The listing builds one solid part. Answer for the finished solid, in the listing's coordinates (mm). Round coordinates to 2 decimals unless told otherwise and drop trailing zeros. Order: outer loops, then holes, each group sorted by start corner. A loop starts at its lowest first (then second) coordinate and runs counter-clockwise, first axis right, second up. Notation, with made-up numbers: (46.25, -37.5) -> (65.25, -37.5) arc R20 ccw to (65.25, -22.5) -> close; hole circle Ø8 at (11.25, -12). An arc over 180 degrees is marked (long way). Return JSON: item names as keys, results as strings. Group by question number.
(1) The part is cut by section B-B (z = -63.5). Determine the outline of the cut face in (x, y).
(2) The part is cut by section A-A (x = -12.7). Determine the outline of the cut face in (y, z).
(3) The part is cut by section D-D (x = -63.5). Determine the outline of the cut face in (y, z), plus the area to 3 significant figures.
(4) The part is cut by section C-C (y = 2). Determine the outline of the cut face in (x, z).
(5) Consider line 1 (Z direction, x = -12.7, y = 4.5); line 2 (Z direction, x = -63.5, y = 5); line 3 (Z direction, x = -51, y = 3.5). Determine where each line is inside the solid, lowest interval first. Write a range as [from, to].
(6) Each of these flat-tipped pins is pushed along its axis until it touches: pin 1 (3 mm diameter, centred on x = -38, y = 0.5, fed in from -Z); pin 2 (4.5 mm diameter, centred on x = -12.7, z = -12.7, fed in from +Y); pin 3 (2 mm diameter, centred on x = -56.5, y = 3.5, fed in from -Z). Where does it stop, or does it pass through?
Autodesk Inventor part; units mm, degrees
ref_plane "YZ Plane" through (0, 0, 0) normal (1, 0, 0) x (0, 1, 0)
ref_plane "XZ Plane" through (0, 0, 0) normal (0, 1, 0) x (-1, 0, 0)
ref_plane "XY Plane" through (0, 0, 0) normal (0, 0, 1) x (1, 0, 0)
sketch "Sketch1" plane through (0, 0, 0) normal (0, 1, 0) x (-1, 0, 0)
  line L0 (0, 0) -> (76.2, 0)
  line L1 (76.2, 0) -> (76.2, -25.4)
  line L2 (76.2, -25.4) -> (50.8, -25.4)
  line L3 (0, -25.4) -> (0, 0)
  line L4 (0, 0) -> (25.4, 0)
  line L5 (25.4, -50.8) -> (25.4, -76.2)
  line L6 (25.4, -76.2) -> (0, -76.2)
  line L7 (0, -76.2) -> (0, 0)
  arc A0 (50.8, -25.4) -> (25.4, -50.8) centre (50.8, -50.8) ccw
  circle A1 centre (63.5, -12.7) radius 2.5
  circle A2 centre (38.1, -12.7) radius 2.5
  circle A3 centre (12.7, -12.7) radius 2.5
  circle A4 centre (12.7, -38.1) radius 2.5
  circle A5 centre (12.7, -63.5) radius 2.5
  point P0 (12.7, -76.2)
  point P1 (76.2, -12.7)
  dimension "d0" = 76.2
  dimension "d1" = 25.4
  dimension "d2" = 25.4
  dimension "d3" = 76.2
  dimension "d4" = 25.4
  dimension "d5" = 5
  dimension "d6" = 5
  dimension "d7" = 5
  dimension "d8" = 5
  dimension "d9" = 5
  dimension "d10" = 12.7
  dimension "d11" = 12.7
  dimension "d12" = 12.7
  dimension "d13" = 12.7
  dimension "d14" = 12.7
  dimension "d15" = 12.7
  dimension "d16" = 38.1
  dimension "d17" = 38.1
  dimension "d18" = 12.7
  dimension "d19" = 12.7
extrude "Extrusion1" add sketch "Sketch1" along normal blind 6.35
equation "\"d12\" = d10"
equation "\"d13\" = d10"
equation "\"d14\" = d10"
equation "\"d15\" = d14"
equation "\"d16\" = 0.5 * d3"
equation "\"d17\" = 0.5 * d0"
equation "\"d18\" = d10"
equation "\"d19\" = d10"
properties part number "90CornerBracket" material "Phenolic Resin"
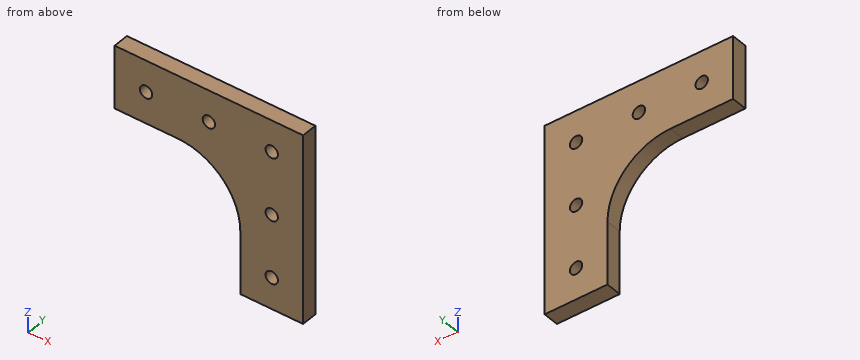
Answer below:
{
 "1": {"outline": "(-25.4, 0) -> (-15.2, 0) -> (-15.2, 6.35) -> (-25.4, 6.35) -> close; (-10.2, 0) -> (0, 0) -> (0, 6.35) -> (-10.2, 6.35) -> close"},
 "2": {"outline": "(0, -76.2) -> (6.35, -76.2) -> (6.35, -66) -> (0, -66) -> close; (0, -61) -> (6.35, -61) -> (6.35, -40.6) -> (0, -40.6) -> close; (0, -35.6) -> (6.35, -35.6) -> (6.35, -15.2) -> (0, -15.2) -> close; (0, -10.2) -> (6.35, -10.2) -> (6.35, 0) -> (0, 0) -> close"},
 "3": {"outline": "(0, -25.4) -> (6.35, -25.4) -> (6.35, -15.2) -> (0, -15.2) -> close; (0, -10.2) -> (6.35, -10.2) -> (6.35, 0) -> (0, 0) -> close", "area": "130 mm²"},
 "4": {"outline": "(-76.2, -25.4) -> (-50.8, -25.4) arc R25.4 cw to (-25.4, -50.8) -> (-25.4, -76.2) -> (0, -76.2) -> (0, 0) -> (-76.2, 0) -> close; hole circle Ø5 at (-63.5, -12.7); hole circle Ø5 at (-38.1, -12.7); hole circle Ø5 at (-12.7, -63.5); hole circle Ø5 at (-12.7, -38.1); hole circle Ø5 at (-12.7, -12.7)"},
 "5": {"line 1": "z = [-76.2, -66], [-61, -40.6], [-35.6, -15.2], [-10.2, 0]", "line 2": "z = [-25.4, -15.2], [-10.2, 0]", "line 3": "z = [-25.4, 0]"},
 "6": {"pin 1": "stops at z = -29.81", "pin 2": "passes through", "pin 3": "stops at z = -25.4"}
}
